For this review, take the finished solid that the model builds, in its own axes (mm). Face numbers are marked on the shaded views. A direction names the side the tool comes from. Coordinates: 2 decimals unless noted, no trailing zeros. Write each loop counter-clockwise with the first axis right and the second up, starting at its lowest first coordinate (ties: lowest second). Pieces come first, ordered by that corner, then holes. Notation, with made-up numbers: M 26.5,40 L 55.5,40 A32 cw 55.5,72 Z; hole C 4,4.5 d1. An arc over 180 degrees is marked long. One line per question, with ' | ' between items.
from build123d import *

# Parameters (mm, degrees)
BOSS_EXTRUDE1_DEPTH = 101.6
SKETCH2_R           = 3.175
CUT_EXTRUDE1_DEPTH  = 203.593055017
SKETCH3_R           = 3.175
CUT_EXTRUDE2_DEPTH  = 203.593055017
SKETCH4_R           = 3.175
CUT_EXTRUDE3_DEPTH  = 179.810196235


with BuildPart() as part:
    # Model → Boss-Extrude1 (new body)
    with BuildSketch(Plane.XY):
        Polygon((93.173661033, 113.358492063), (97.136061033, 117.320892063), (147.936061033, 117.320892063), (151.898461033, 113.358492063), (151.898461033, 90.346092063), (155.860861033, 90.346092063), (155.860861033, 113.358492063), (172.523261033, 113.358492063), (172.523261033, 121.283292063), (72.548861033, 121.283292063), (72.548861033, 113.358492063), (89.211261033, 113.358492063), (89.211261033, 90.346092063), (93.173661033, 90.346092063), align=None)
    extrude(amount=BOSS_EXTRUDE1_DEPTH)

    # Sketch2 → Cut-Extrude1 (cut, through all)
    with BuildSketch(Plane(origin=(0, 121.283292063, 0), x_dir=(1, 0, 0), z_dir=(0, 1, 0))):
        with Locations(Location((163.811061033, -12.7, 0), (0, 0, 270))):
            Circle(SKETCH2_R)
        with Locations(Location((163.811061033, -38.1, 0), (0, 0, 270))):
            Circle(SKETCH2_R)
        with Locations(Location((163.811061033, -63.5, 0), (0, 0, 270))):
            Circle(SKETCH2_R)
        with Locations(Location((163.811061033, -88.9, 0), (0, 0, 270))):
            Circle(SKETCH2_R)
        with Locations(Location((81.261061033, -38.1, 0), (0, 0, 270))):
            Circle(SKETCH2_R)
        with Locations(Location((81.261061033, -63.5, 0), (0, 0, 270))):
            Circle(SKETCH2_R)
        with Locations(Location((81.261061033, -88.9, 0), (0, 0, 270))):
            Circle(SKETCH2_R)
        with Locations(Location((81.261061033, -12.7, 0), (0, 0, 270))):
            Circle(SKETCH2_R)
    extrude(amount=-CUT_EXTRUDE1_DEPTH, mode=Mode.SUBTRACT)

    # Sketch3 → Cut-Extrude2 (cut, through all)
    with BuildSketch(Plane(origin=(0, 121.283292063, 0), x_dir=(1, 0, 0), z_dir=(0, 1, 0))):
        with Locations(Location((135.236061033, -25.4, 0), (0, 0, 270))):
            Circle(SKETCH3_R)
        with Locations(Location((109.836061033, -25.4, 0), (0, 0, 270))):
            Circle(SKETCH3_R)
        with Locations(Location((109.836061033, -76.2, 0), (0, 0, 270))):
            Circle(SKETCH3_R)
        with Locations(Location((135.236061033, -76.2, 0), (0, 0, 270))):
            Circle(SKETCH3_R)
    extrude(amount=-CUT_EXTRUDE2_DEPTH, mode=Mode.SUBTRACT)

    # Sketch4 → Cut-Extrude3 (cut, through all)
    with BuildSketch(Plane.ZY.offset(-89.211261033)):
        with Locations((25.4, 99.871092063)):
            Circle(SKETCH4_R)
        with Locations((76.2, 99.871092063)):
            Circle(SKETCH4_R)
    extrude(amount=-CUT_EXTRUDE3_DEPTH, mode=Mode.SUBTRACT)


solid = part.part
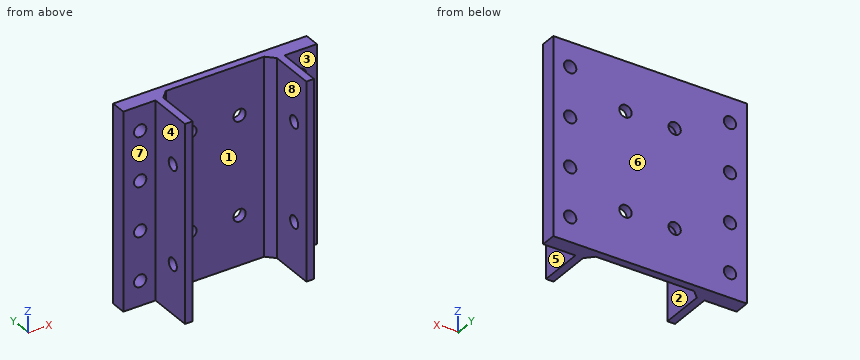
1) To check wall thickness, follow line 1 along X through (y, z) = (118.5, 12.7); line 2 along X through (y, z) = (120, 76); line 3 along X through (y, z) = (104.5, 84). State the ranges of each line that lie inside material, in increasing order. Write a range as [from, to].
Responses:
line 1: [72.55, 78.09], [84.44, 160.64], [166.99, 172.52] | line 2: [72.55, 106.67], [113, 132.07], [138.4, 172.52] | line 3: [89.21, 93.17], [151.9, 155.86]
2) We need section A-A on y = 108.5. State the section outline as (x, z) points, then the cut area to 3 significant figures.
Responses:
outline: M 89.21,0 L 93.17,0 L 93.17,101.6 L 89.21,101.6 Z; M 151.9,0 L 155.86,0 L 155.86,101.6 L 151.9,101.6 Z | area: 805 mm^2
3) We need section C-C on z = 63.5. State the section outline as (x, y) points, then the cut area to 3 significant figures.
Responses:
outline: M 72.55,113.36 L 78.09,113.36 L 78.09,121.28 L 72.55,121.28 Z; M 84.44,113.36 L 89.21,113.36 L 89.21,90.35 L 93.17,90.35 L 93.17,113.36 L 97.14,117.32 L 147.94,117.32 L 151.9,113.36 L 151.9,90.35 L 155.86,90.35 L 155.86,113.36 L 160.64,113.36 L 160.64,121.28 L 84.44,121.28 Z; M 166.99,113.36 L 172.52,113.36 L 172.52,121.28 L 166.99,121.28 Z | area: 657 mm^2
4) The part is to be moulded in two halves that separate along X. For the marked faces 1, 2, 3 and 4, say which applies: +X half, -X half, draft (parallel to the pull), parting line (faces both ways), or undercut.
Responses:
face 1: undercut | face 2: undercut | face 3: draft | face 4: -X half
5) We need section B-B on z = 76.2. State how many separate pieces and enclosed holes the cut face has, then the cut area to 3 significant figures.
Responses:
separate pieces: 5 | enclosed holes: 0 | area: 657 mm^2
6) Insertion check: pin 1 Ø8 at (y, z) = (102.5, 65.5) entering from -X; pin 2 Ø10 at (x, z) = (131.5, 90) entering from -Y; pin 3 Ø11.5 at (y, z) = (98, 29.5) entering from +X; pin 4 Ø10 at (x, y) = (101, 94) entering from -Z. Each pin has a flat end and moves straight along its axis. Give the tip position at first contact, or say it passes through.
Responses:
pin 1: x = 89.21 | pin 2: y = 117.32 | pin 3: x = 155.86 | pin 4: through
7) Machinability: for the marked faces 5, 6, 7 and 8, which of the approach directions +Z, -Z, +X, -X, +Y, -Y give a long, thin tool a straight path to every point of the face, cutting with its end or side? Answer none if there is none.
Responses:
face 5: +Z, -Z, +X, -Y | face 6: +Z, -Z, +X, -X, +Y | face 7: +Z, -Z, -X, -Y | face 8: +Z, -Z, -Y
8) We need section D-D on z = 30. State the section outline as (x, y) points, then the cut area to 3 significant figures.
Responses:
outline: M 72.55,113.36 L 89.21,113.36 L 89.21,90.35 L 93.17,90.35 L 93.17,113.36 L 97.14,117.32 L 147.94,117.32 L 151.9,113.36 L 151.9,90.35 L 155.86,90.35 L 155.86,113.36 L 172.52,113.36 L 172.52,121.28 L 72.55,121.28 Z | area: 758 mm^2
